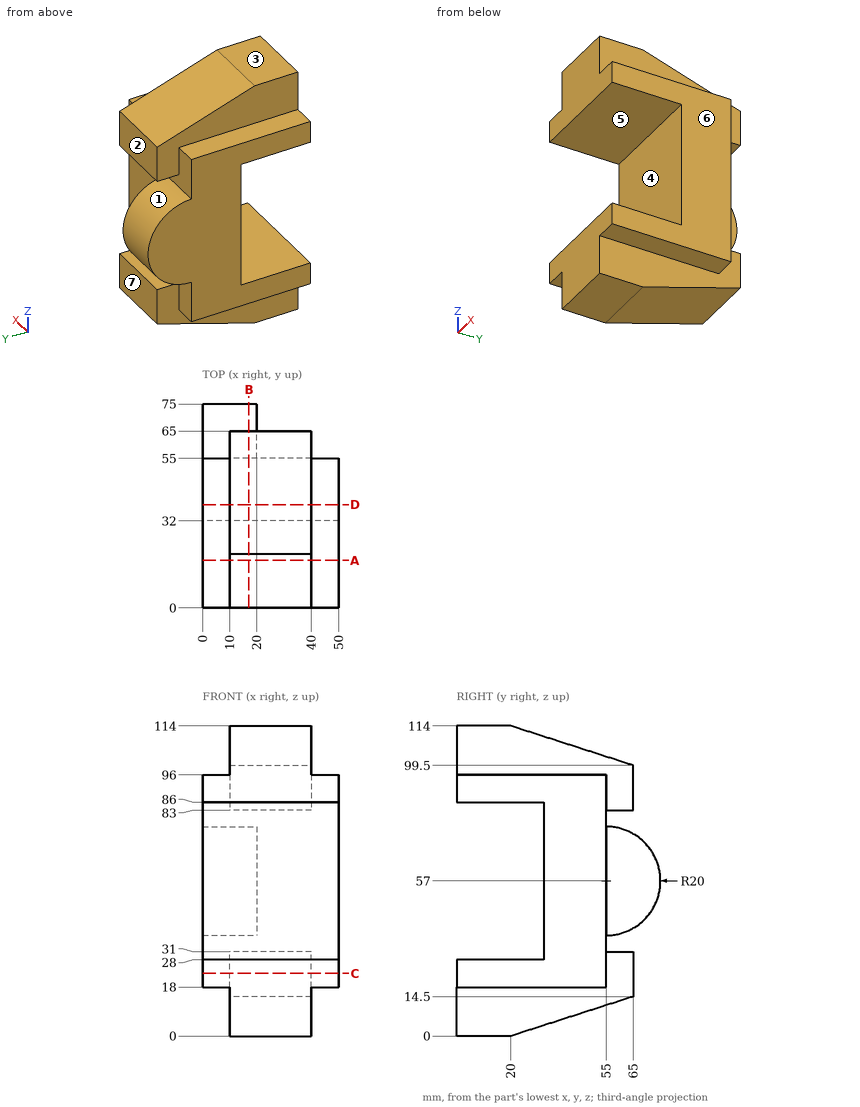
Input: dimensioned drawing with shaded views. Units: mm. Origin: part minimum x, y, z. A direction names the side the tool comes from. Coordinates: 2 decimals unless noted, no trailing zeros. Order: outer loops, then holes, each group sorted by start corner. A loop starts at its lowest first (then second) coordinate and runs counter-clockwise, first axis right, second up. Notation, with made-up numbers: (80.25, 70) -> (121.25, 70) arc R24 cw to (121.25, 84) -> close; hole circle Ø8 at (12, -28). An arc over 180 degrees is marked (long way). Answer in a Markdown table with one row per item.
Item 1: Draft query along Z for the marked faces 1, 2, 3 and 4. Return one class per face: released by +Z, released by -Z, zero draft, split by the parting line, or undercut.
Return value:
| item | result |
|---|---|
| face 1 | undercut |
| face 2 | zero draft |
| face 3 | released by +Z |
| face 4 | undercut |
Item 2: Ray query, L1, parallel to Z at x = 14, y = 19; L2, parallel to Y at x = 8.5, z = 81; L3, parallel to X at y = 56.5, z = 21. Return the intervals inside material, ascending.
Return value:
| item | result |
|---|---|
| L1 | z = 0 to 28, 86 to 114 |
| L2 | y = 32 to 55 |
| L3 | x = 10 to 40 |
Item 3: Access query for the marked faces 5, 6 and 7. Directions: +Z, -Z, +X, -X, +Y, -Y. A direction counts if a zero-diameter tool reaches every point of the face in a straight line with its end or side. Return the directions, or none.
Return value:
| item | result |
|---|---|
| face 5 | +X, -X, -Y |
| face 6 | +Z, -Z, +X, +Y, -Y |
| face 7 | -Z, +X, -X, +Y |
Item 4: Section A-A on y = 17.5. Output: boundary loops of the cut face in (x, z), plus the area to 3 significant figures.
Return value:
| item | result |
|---|---|
| outline | (0, 18) -> (10, 18) -> (10, 0) -> (40, 0) -> (40, 18) -> (50, 18) -> (50, 28) -> (0, 28) -> close; (0, 86) -> (50, 86) -> (50, 96) -> (40, 96) -> (40, 114) -> (10, 114) -> (10, 96) -> (0, 96) -> close |
| area | 2,080 mm² |
Item 5: Section D-D on y = 38. Output: boundary loops of the cut face in (x, z).
Return value:
| item | result |
|---|---|
| outline | (0, 18) -> (10, 18) -> (10, 5.8) -> (40, 5.8) -> (40, 18) -> (50, 18) -> (50, 96) -> (40, 96) -> (40, 108.2) -> (10, 108.2) -> (10, 96) -> (0, 96) -> close |
Item 6: Contact query for flat-ended pins moving along their axis: P1, Ø1, axis at x = 19, y = 25, coming from the +Z side; P2, Ø5, axis at x = 37.5, z = 69, coming from the -Y side; P3, Ø3, axis at y = 30, z = 46, coming from the +X side; P4, Ø4, axis at x = 20, z = 34.5, coming from the +Y side. Output: stop coordinate, or through.
Return value:
| item | result |
|---|---|
| P1 | stops at z = 112.55 |
| P2 | stops at y = 32 |
| P3 | passes through |
| P4 | stops at y = 55 |
Item 7: Section B-B on x = 17. Output: boundary loops of the cut face in (y, z), plus the area to 3 significant figures.
Return value:
| item | result |
|---|---|
| outline | (0, 0) -> (20, 0) -> (65, 14.5) -> (65, 31) -> (55, 31) -> (55, 37) arc R20 ccw to (55, 77) -> (55, 83) -> (65, 83) -> (65, 99.5) -> (20, 114) -> (0, 114) -> (0, 86) -> (32, 86) -> (32, 28) -> (0, 28) -> close |
| area | 5,010 mm² |
Item 8: Section C-C on z = 23. Output: boundary loops of the cut face in (x, y).
Return value:
| item | result |
|---|---|
| outline | (0, 0) -> (50, 0) -> (50, 55) -> (40, 55) -> (40, 65) -> (10, 65) -> (10, 55) -> (0, 55) -> close |
